Part print with two shaded views. Sizes in mm from the minimum x, y, z corner. A direction names the side the tool comes from. Coordinates: 2 decimals unless noted, no trailing zeros. Loops run counter-clockwise (first coordinate to the right, second up) from the corner with the lowest first, then second, coordinate; pieces in that order, holes last.
(1) Wall check: L1, parallel to Z at x = 34.1, y = 1.35 (3 decimals); L2, parallel to X at y = 0.7, z = 94.55; L3, parallel to Z at x = 34, y = 1 (3 decimals). Give the ranges that are in metal, low to high.
(2) Slice it at A-A (z = 45). Give the cut face in (x, y) (3 decimals).
(3) Slice it at C-C (y = 23.5). Give the cut face in (x, z) (3 decimals), and give its area (3 significant figures).
(4) Slice it at B-B (x = 25). Give the cut face in (y, z) (3 decimals), and give its area (3 significant figures).
(5) Two-plate mould, pull along Z, no slides. Class the marked faces 6, 7 and 8: pulls with the +Z half, pulls with the -Z half, needs draft (parallel to the pull), parting line crosses it, or undercut.
(6) Tool access for the marked faces 1, 2, 3, 4 and 5: list every direction of +Z, -Z, +X, -X, +Y, -Y with a clear straight run to the whole face (end or side of a thin tool).
(7) Flat gauge pins, fed straight in: P1, Ø2.5, axis at x = 34.1, z = 4, coming from the +Y side; P2, Ø5, axis at x = 26.5, y = 27.5, coming from the +Z side; P3, Ø5, axis at x = 4, y = 25, coming from the -Z side; P4, Ø2.5, axis at x = 25, z = 2, coming from the +Y side. Where does each tip first touch, or does it go through?
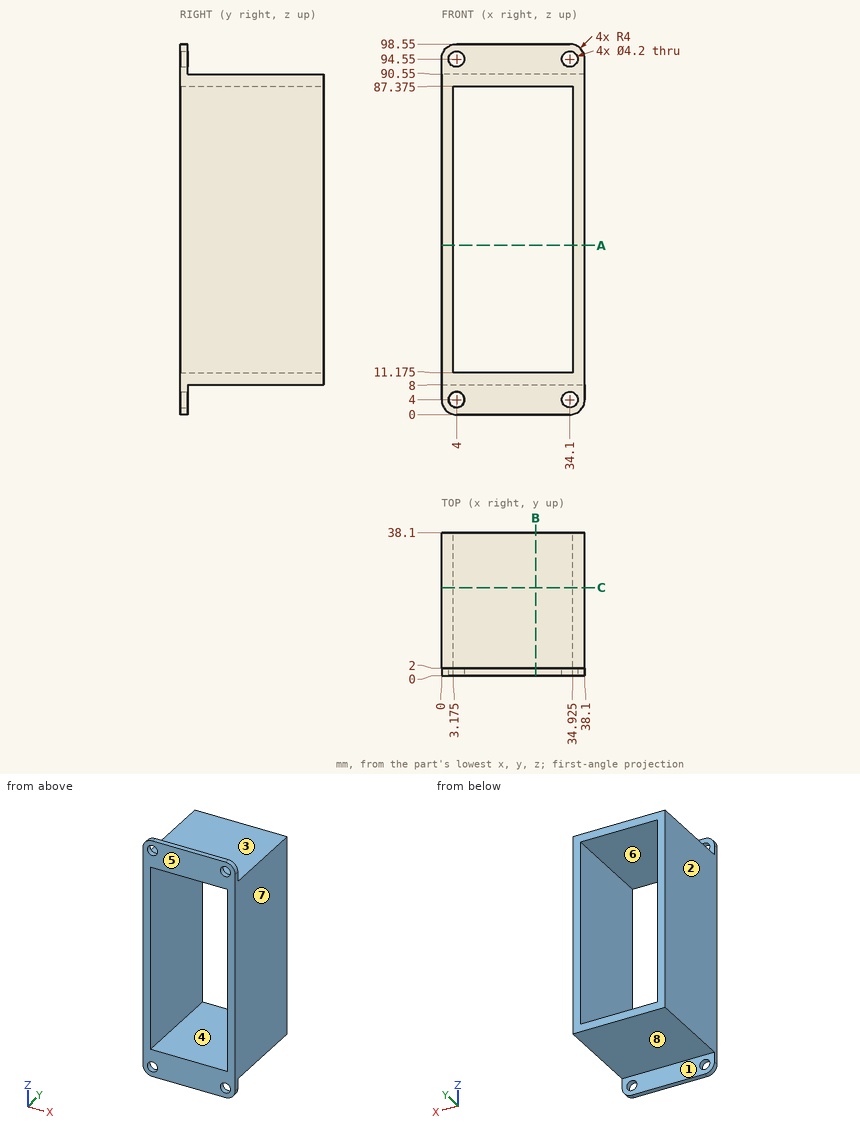
Response values:
1. L1: z = 0 to 1.9, 6.1 to 11.175, 87.375 to 92.45, 96.65 to 98.55
1. L2: x = 0 to 1.9, 6.1 to 32, 36.2 to 38.1
1. L3: z = 0 to 1.902, 6.098 to 11.175, 87.375 to 92.452, 96.648 to 98.55
2. outline: (0, 0) - (3.175, 0) - (3.175, 38.1) - (0, 38.1) - close; (34.925, 0) - (38.1, 0) - (38.1, 38.1) - (34.925, 38.1) - close
3. outline: (0, 8) - (38.1, 8) - (38.1, 90.55) - (0, 90.55) - close; hole (3.175, 11.175) - (34.925, 11.175) - (34.925, 87.375) - (3.175, 87.375) - close
3. area: 726 mm2
4. outline: (0, 0) - (2, 0) - (2, 8) - (38.1, 8) - (38.1, 11.175) - (0, 11.175) - close; (0, 87.375) - (38.1, 87.375) - (38.1, 90.55) - (2, 90.55) - (2, 98.55) - (0, 98.55) - close
4. area: 274 mm2
5. face 6: undercut
5. face 7: needs draft
5. face 8: pulls with the -Z half
6. face 1: -Z, +X, -X, +Y
6. face 2: +Z, -Z, -X, +Y, -Y
6. face 3: +Z, +X, -X, +Y
6. face 4: +Y, -Y
6. face 5: +Z, -Z, +X, -X, -Y
7. P1: passes through
7. P2: stops at z = 90.55
7. P3: stops at z = 8
7. P4: stops at y = 2
